```python
from build123d import *

# Parameters (mm, degrees)
SKETCH1_R                = 40
SKETCH1_R_2              = 10
BOSS_EXTRUDE1_DEPTH      = 12.5
SKETCH2_R                = 22.5
CUT_EXTRUDE1_DEPTH       = 10
SKETCH3_R                = 4
CUT_EXTRUDE2_DEPTH       = 16
CIRPATTERN1_COUNT        = 5
SKETCH4_R                = 11
SKETCH4_R_2              = 10
BOSS_EXTRUDE2_DEPTH      = 2
BOSS_EXTRUDE2_DEPTH_BACK = 7


with BuildPart() as part:
    # Sketch1 → Boss-Extrude1 (new body, symmetric)
    with BuildSketch(Plane.XY):
        Circle(SKETCH1_R)
        Circle(SKETCH1_R_2, mode=Mode.SUBTRACT)
    extrude(amount=BOSS_EXTRUDE1_DEPTH, both=True)

    # Sketch2 → Cut-Extrude1 (cut)
    with BuildSketch(Plane.XY.offset(12.5)):
        Circle(SKETCH2_R)
    cut_extrude1 = extrude(amount=-CUT_EXTRUDE1_DEPTH, mode=Mode.SUBTRACT)

    # Mirror1: Cut-Extrude1 across plane
    add(cut_extrude1.mirror(Plane.XY), mode=Mode.SUBTRACT)

    # Sketch3 → Cut-Extrude2 (cut, through all)
    with BuildSketch(Plane.XY.offset(2.5)):
        with Locations((0, 17)):
            Circle(SKETCH3_R)
    cut_extrude2 = extrude(amount=-CUT_EXTRUDE2_DEPTH, mode=Mode.SUBTRACT)

    # CirPattern1: Cut-Extrude2 ×5 about axis
    cirpattern1_axis = Axis((0, 0, 0), (0, 0, 1))
    for i in range(1, CIRPATTERN1_COUNT):
        add(cut_extrude2.rotate(cirpattern1_axis, i * 360 / CIRPATTERN1_COUNT), mode=Mode.SUBTRACT)

    # Sketch4 → Boss-Extrude2 (add, two sides)
    with BuildSketch(Plane.XY.offset(2.5)) as boss_extrude2_sk:
        Circle(SKETCH4_R)
        Circle(SKETCH4_R_2, mode=Mode.SUBTRACT)
    extrude(amount=BOSS_EXTRUDE2_DEPTH)
    extrude(boss_extrude2_sk.sketch, amount=-BOSS_EXTRUDE2_DEPTH_BACK)

    # Sketch5 → Cut-Revolve1 (revolve, cut)
    with BuildSketch(Plane(origin=(0, 0, 0), x_dir=(1, 0, 0), z_dir=(0, 1, 0))):
        Polygon((-40, 9.5), (-40, -9.5), (-34, -6.036086587), (-34, 6.035898385), align=None)
    revolve(axis=Axis((0, 0, 0), (0, 0, -1)), mode=Mode.SUBTRACT)


solid = part.part
```
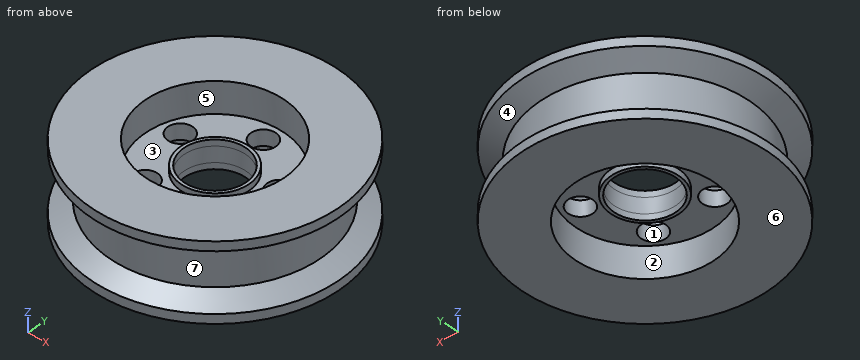
For this review, take the finished solid that the model builds, in its own axes (mm). Face numbers are marked on the shaded views. A direction names the side the tool comes from. Give positions to 0.01 mm unless a question says otherwise; leave off trailing zeros. Order: outer loops, then holes, each group sorted by start corner. A loop starts at its lowest first (then second) coordinate and runs counter-clockwise, first axis right, second up.
1) Take a section at C-C (x = 0). State how many separate pieces and enclosed holes the cut face has, then the cut area to 3 significant figures.
2) Take a section at B-B (z = 1.5). Give the boundary of the cut face in (x, y).
3) Insertion check: pin 1 (1.5 mm diameter, centred on y = -2.5, z = 6, fed in from -X); pin 2 (12 mm diameter, centred on y = 0.5, z = 9, fed in from -X); pin 3 (5 mm diameter, centred on y = 21.5, z = -5.5, fed in from +X); pin 4 (9 mm diameter, centred on x = 9.99, y = -13.75, fed in from +Z). Each pin has a flat end and moves straight along its axis. Give the tip position at first contact, or say it passes through.
4) The part is to be moulded in two halves that separate along Y. For the marked faces 5, 6 and 7, say which applies: released by +Y, released by -Y, zero draft, split by the parting line, or undercut.
5) For the marked faces 1, 2, 3 and 4, list the 3-axis set-ups (+Z, -Z, +X, -X, +Y, -Y) from which the entire face can be reached by the end or side of a thin tool; tool diameter is ignored.
6) Take a section at D-D (z = -7). Give the boundary of the cut face in (x, y), then the cut area to 3 significant figures.
7) Wall thickness on line 1 (Y direction, x = 0, z = 3.05); line 2 (X direction, y = -0.5, z = 3); line 3 (Y direction, x = 0, z = 6): over which ranges is each line inside the solid? List them lowest first.
Derived:
1. separate pieces: 3
1. enclosed holes: 0
1. area: 782 mm2
2. outline: circle Ø68 at (0, 0); hole circle Ø8 at (-16.17, 5.25); hole circle Ø8 at (-9.99, -13.75); hole circle Ø20 at (0, 0); hole circle Ø8 at (0, 17); hole circle Ø8 at (9.99, -13.75); hole circle Ø8 at (16.17, 5.25)
3. pin 1: stops at x = -35.15
3. pin 2: stops at x = -40
3. pin 3: stops at x = 30.88
3. pin 4: stops at z = 2.5
4. face 5: undercut
4. face 6: zero draft
4. face 7: split by the parting line
5. face 1: +Z, -Z
5. face 2: -Z
5. face 3: +Z
5. face 4: none
6. outline: circle Ø71.34 at (0, 0); hole circle Ø45 at (0, 0)
6. area: 2,410 mm2
7. line 1: y = -34 to -22.5, -11 to -10, 10 to 11, 22.5 to 34
7. line 2: x = -34 to -22.49, -10.99 to -9.99, 9.99 to 10.99, 22.49 to 34
7. line 3: y = -34 to -22.5, 22.5 to 34
